Source: three-view drawing plus pictorial views. Frame: mm from the lowest corner of the part. Give positions to 0.01 mm unless a question says otherwise; leave off trailing zeros. Order: outer loops, then holes, each group sorted by start corner. A loop starts at its lowest first (then second) coordinate and runs counter-clockwise, first axis right, second up. Notation, with made-up numbers: (-26, 68) -> (33, 68) arc R19 cw to (33, 87) -> close; hole circle Ø7 at (-3.75, 28.5). An arc over 180 degrees is marked (long way). Use a Markdown table: item, result. Add a question column.
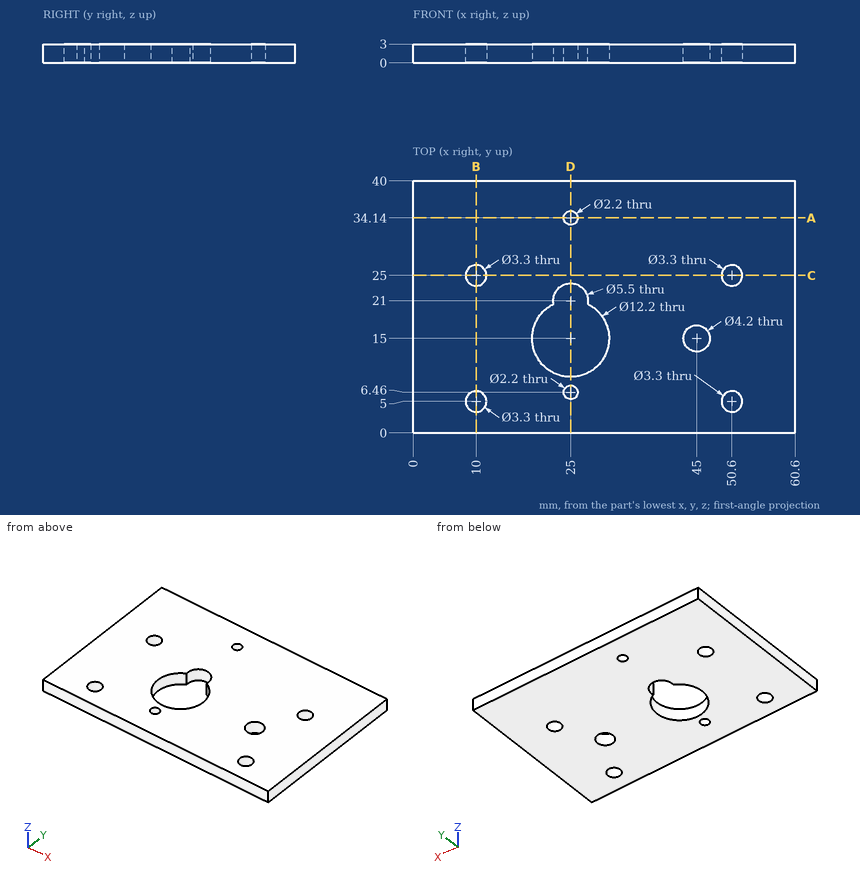
Q1. Ray query, line 1 (Y direction, x = 10, z = 1.3); line 2 (Y direction, x = 26, z = 0.3); line 3 (Y direction, x = 24.5, z = 0.9). Return the intervals inside material, ascending.
Q2. Section query D-D (x = 25). Return loops of the section in (y, z).
Q3. Section query A-A (y = 34.14). Return loops of the section in (x, z).
Q4. Section query B-B (x = 10). Return loops of the section in (y, z), plus the area to 3 significant figures.
Q5. First-contact query: pin 1 (1.3 mm diameter, centred on x = 25, y = 6.46, fed in from +Z). Flat tip, straight axial feed; report the tip coordinate or a pass-through.
Q6. Section query C-C (y = 25). Return loops of the section in (x, z), plus the area to 3 significant figures.
Solution:
| question | item | result |
|---|---|---|
| 1 | line 1 | y = 0 to 3.35, 6.65 to 23.35, 26.65 to 40 |
| 1 | line 2 | y = 0 to 6, 6.92 to 8.98, 23.56 to 33.68, 34.6 to 40 |
| 1 | line 3 | y = 0 to 5.48, 7.44 to 8.92, 23.7 to 33.16, 35.12 to 40 |
| 2 | outline | (0, 0) -> (5.36, 0) -> (5.36, 3) -> (0, 3) -> close; (7.56, 0) -> (8.9, 0) -> (8.9, 3) -> (7.56, 3) -> close; (23.75, 0) -> (33.04, 0) -> (33.04, 3) -> (23.75, 3) -> close; (35.24, 0) -> (40, 0) -> (40, 3) -> (35.24, 3) -> close |
| 3 | outline | (0, 0) -> (23.9, 0) -> (23.9, 3) -> (0, 3) -> close; (26.1, 0) -> (60.6, 0) -> (60.6, 3) -> (26.1, 3) -> close |
| 4 | outline | (0, 0) -> (3.35, 0) -> (3.35, 3) -> (0, 3) -> close; (6.65, 0) -> (23.35, 0) -> (23.35, 3) -> (6.65, 3) -> close; (26.65, 0) -> (40, 0) -> (40, 3) -> (26.65, 3) -> close |
| 4 | area | 100 mm² |
| 5 | pin 1 | passes through |
| 6 | outline | (0, 0) -> (8.35, 0) -> (8.35, 3) -> (0, 3) -> close; (11.65, 0) -> (48.95, 0) -> (48.95, 3) -> (11.65, 3) -> close; (52.25, 0) -> (60.6, 0) -> (60.6, 3) -> (52.25, 3) -> close |
| 6 | area | 162 mm² |
